```python
from build123d import *

# Parameters (mm, degrees)
SKETCH1_W           = 77.47
SKETCH1_H           = 127
BOSS_EXTRUDE1_DEPTH = 11.43
SKETCH2_R           = 3.175
CUT_EXTRUDE1_DEPTH  = 128
CUT_EXTRUDE2_DEPTH  = 12.43
SKETCH4_W           = 54.61
SKETCH4_H           = 6.35
CUT_EXTRUDE3_DEPTH  = 128
CHAMFER1_SIZE       = 2.54


with BuildPart() as part:
    # Sketch1 → Boss-Extrude1 (new body)
    with BuildSketch(Plane(origin=(0, 0, 0), x_dir=(1, 0, 0), z_dir=(0, 1, 0))):
        with Locations((38.735, 63.5)):
            Rectangle(SKETCH1_W, SKETCH1_H)
    extrude(amount=BOSS_EXTRUDE1_DEPTH)

    # Sketch2 → Cut-Extrude1 (cut, through all)
    with BuildSketch(Plane.XY):
        with Locations((5.715, 5.715)):
            Circle(SKETCH2_R)
        with Locations((71.755, 5.715)):
            Circle(SKETCH2_R)
    extrude(amount=-CUT_EXTRUDE1_DEPTH, mode=Mode.SUBTRACT)

    # Sketch3 → Cut-Extrude2 (cut, through all)
    with BuildSketch(Plane(origin=(0, 11.43, 0), x_dir=(1, 0, 0), z_dir=(0, 1, 0))):
        with BuildLine():
            Line((11.43, 127), (11.43, 88.9))
            ThreePointArc((11.43, 88.9), (15.149743879, 79.919743879), (24.13, 76.2))
            Line((24.13, 76.2), (53.34, 76.2))
            ThreePointArc((53.34, 76.2), (62.320256121, 79.919743879), (66.04, 88.9))
            Line((66.04, 88.9), (66.04, 127))
            Line((66.04, 127), (11.43, 127))
        make_face()
    extrude(amount=-CUT_EXTRUDE2_DEPTH, mode=Mode.SUBTRACT)

    # Sketch4 → Cut-Extrude3 (cut, through all)
    with BuildSketch(Plane(origin=(0, 0, -127), x_dir=(-1, 0, 0), z_dir=(0, 0, -1))):
        with Locations((-38.735, 8.255)):
            Rectangle(SKETCH4_W, SKETCH4_H)
    extrude(amount=-CUT_EXTRUDE3_DEPTH, mode=Mode.SUBTRACT)

    # Chamfer1
    chamfer1_edges = [part.edges().sort_by_distance(p)[0] for p in [
        (77.47, 11.43, -63.5),
        (0, 11.43, -63.5),
        (77.47, 0, -63.5),
        (0, 0, -63.5),
    ]]
    chamfer(chamfer1_edges, length=CHAMFER1_SIZE)


solid = part.part
```
Can you work these out from the model? Positions are in its coordinate system, mm. A direction names the side the tool comes from. Round coordinates to 2 decimals unless told otherwise and drop trailing zeros. Loops run counter-clockwise (first coordinate to the right, second up) from the corner with the lowest first, then second, coordinate; pieces in that order, holes last. Notation, with made-up numbers: M -25.75,56.5 L 26.25,56.5 A23 cw 26.25,94.5 Z; hole C 79.5,46.5 d11. An arc over 180 degrees is marked long. Write item = value, one per line. Start each with the question number.
(1) Which directions (+Z, -Z, +X, -X, +Y, -Y) give clear straight access to the entire face, cutting with the end or side of a thin tool? Please do faces 4 (the face through (39, 5.08, -35)), 5 (the face through (15.05, 2.58, -80.02)), 6 (the face through (1.29, 10.18, -62.61)), 7 (the face through (11.43, 7, -79)).
(2) I need wall thicknesses on line 1 along X through (y, z) = (6.5, -117.5); line 2 along X through (y, z) = (5.25, -103); line 3 along X through (y, z) = (4.5, -47). Which ranges of each line are inside material? Lowest first, please.
(3) Suppose I cut it at D-D on x = 29. Write out the boundary of the cut face in (y, z), plus the area to 3 significant figures.
(4) I'm going to push a flat-ended pin straight in: P1, Ø4, axis at x = 36, y = 3.5, coming from the -Z side. Where does the tip first touch, or does it pass through?
(5) Suppose I cut it at C-C on z = -25.5. Write out the boundary of the cut face in (x, y) (3 decimals), plus the area to 3 significant figures.
(6) Suppose I cut it at A-A on z = -112.5. Write out the boundary of the cut face in (x, y) (3 decimals), plus the area to 3 significant figures.
(7) Suppose I cut it at B-B on y = 1.25. Write out the boundary of the cut face in (x, z), plus the area to 3 significant figures.
(8) If we mould it in two halves opening along Y, with no side actions, what happens to faces 1 (the face through (5.027, 2.616, -62.611)), 2 (the face through (7, 11.43, -64)), 3 (the face through (62.2, 2.6, -79.8))? For each: released by +Y, released by -Y, zero draft, split by the parting line, or undercut.
Answer block:
q1.face_4 = +Z, -Z, +Y
q1.face_5 = -Z, +Y, -Y
q1.face_6 = +Z, -Z, -X, +Y
q1.face_7 = -Z, +Y
q2.line_1 = 0 to 2.64, 8.79 to 11.43, 66.04 to 68.68, 74.83 to 77.47
q2.line_2 = 0 to 2.57, 8.86 to 11.43, 66.04 to 68.61, 74.9 to 77.47
q2.line_3 = 0 to 2.78, 8.65 to 68.82, 74.69 to 77.47
q3.outline = M 0,-76.2 L 5.08,-76.2 L 5.08,0 L 0,0 Z
q3.area = 387 mm²
q4.P1 = -76.2
q5.outline = M 0,2.54 L 2.54,0 L 74.93,0 L 77.47,2.54 L 77.47,8.89 L 74.93,11.43 L 66.04,11.43 L 66.04,5.08 L 11.43,5.08 L 11.43,11.43 L 2.54,11.43 L 0,8.89 Z; hole C 5.715,5.715 d6.35; hole C 71.755,5.715 d6.35
q5.area = 462 mm²
q6.outline = M 0,2.54 L 2.54,0 L 11.43,0 L 11.43,11.43 L 2.54,11.43 L 0,8.89 Z; M 66.04,0 L 74.93,0 L 77.47,2.54 L 77.47,8.89 L 74.93,11.43 L 66.04,11.43 Z; hole C 5.715,5.715 d6.35; hole C 71.755,5.715 d6.35
q6.area = 185 mm²
q7.outline = M 1.29,-127 L 11.43,-127 L 11.43,-88.9 A12.7 cw 24.13,-76.2 L 53.34,-76.2 A12.7 cw 66.04,-88.9 L 66.04,-127 L 76.18,-127 L 76.18,0 L 1.29,0 Z
q7.area = 6,810 mm²
q8.face_1 = undercut
q8.face_2 = released by +Y
q8.face_3 = zero draft
